Source: CAD feature listing. Evaluate the final solid. Frame: model axes, mm. A direction names the side the tool comes from. Coordinates: 2 decimals unless noted, no trailing zeros. Order: outer loops, then holes, each group sorted by start corner. A loop starts at its lowest first (then second) coordinate and runs counter-clockwise, first axis right, second up. Notation, with made-up numbers: (-36, -8) - (2, -8) arc R24 cw to (2, 2) - close; hole circle Ø4 at (62, 87.5). An arc over 180 degrees is marked (long way). One line per question, with ' | ' between items. Start each with the question number.
(1) Section A-A (z = -198.5). Return the cut outline in (x, y) (3 decimals), then the cut area to 3 significant figures.
(2) Section B-B (x = 88.5). Return the cut outline in (y, z) (3 decimals).
(3) Line query: line 1 along Z through (x, y) = (24.5, 0.5); line 2 along Z through (x, y) = (128.5, 7); line 3 along X through (y, z) = (5, -198). Output: solid intervals per line, ascending.
(4) Section C-C (y = 2). Count the separate pieces of the cut face and the enclosed holes in it, then the cut area to 3 significant figures.
(5) Draft query along Z for faces 1 (the flat face through (0, 5, -150)), 2 (the flat face through (88, 5, 0)), 3 (the cylindrical face through (19.69, 1.69, -19.59)). Return one class per face: +Z half, -Z half, draft (parallel to the pull), parting line (faces both ways), or undercut.
(6) Contact query for a flat-ended pin moving along its axis: P1, Ø4.5, axis at x = 62.357, z = -4.445, coming from the +Y side. Output: stop coordinate, or through.
(7) Access query for faces 4 (the cylindrical face through (158.11, 1.69, -19.59)), 5 (the cylindrical face through (13.05, 6.64, -13.3)), 6 (the flat face through (16, 0, -176)). Directions: +Z, -Z, +X, -X, +Y, -Y. A direction counts if a zero-diameter tool reaches every point of the face in a straight line with its end or side. Return the directions, or none.
from build123d import *

# Parameters (mm, degrees)
SKETCH1_W           = 177.8
SKETCH1_H           = 304.8
BOSS_EXTRUDE1_DEPTH = 9.525
SKETCH2_W           = 142.24
SKETCH2_H           = 269.24
CUT_EXTRUDE1_DEPTH  = 10.525
SKETCH3_R           = 2.5527
CUT_EXTRUDE2_DEPTH  = 10.525
FILLET4_R           = 6.35
CUT_EXTRUDE5_DEPTH  = 5.842
CHAMFER1_SIZE       = 0.254
FILLET5_R           = 2.54


with BuildPart() as part:
    # Sketch1 → Boss-Extrude1 (new body)
    with BuildSketch(Plane(origin=(0, 0, 0), x_dir=(1, 0, 0), z_dir=(0, 1, 0))):
        with Locations((88.9, 152.4)):
            Rectangle(SKETCH1_W, SKETCH1_H)
    extrude(amount=BOSS_EXTRUDE1_DEPTH)

    # Sketch2 → Cut-Extrude1 (cut, through all)
    with BuildSketch(Plane(origin=(0, 9.525, 0), x_dir=(1, 0, 0), z_dir=(0, 1, 0))):
        with Locations((88.9, 152.4)):
            Rectangle(SKETCH2_W, SKETCH2_H)
    extrude(amount=-CUT_EXTRUDE1_DEPTH, mode=Mode.SUBTRACT)

    # Sketch3 → Cut-Extrude2 (cut, through all)
    with BuildSketch(Plane(origin=(0, 9.525, 0), x_dir=(1, 0, 0), z_dir=(0, 1, 0))):
        with Locations((4.445, 184.15)):
            Circle(SKETCH3_R)
        with Locations((4.445, 241.3)):
            Circle(SKETCH3_R)
        with Locations((62.357, 300.355)):
            Circle(SKETCH3_R)
        with Locations((4.445, 300.355)):
            Circle(SKETCH3_R)
        with Locations((173.355, 184.15)):
            Circle(SKETCH3_R)
        with Locations((173.355, 241.3)):
            Circle(SKETCH3_R)
        with Locations((173.355, 300.355)):
            Circle(SKETCH3_R)
        with Locations((115.443, 300.355)):
            Circle(SKETCH3_R)
        with Locations((173.355, 120.65)):
            Circle(SKETCH3_R)
        with Locations((173.355, 63.5)):
            Circle(SKETCH3_R)
        with Locations((173.355, 4.445)):
            Circle(SKETCH3_R)
        with Locations((115.443, 4.445)):
            Circle(SKETCH3_R)
        with Locations((62.357, 4.445)):
            Circle(SKETCH3_R)
        with Locations((4.445, 4.445)):
            Circle(SKETCH3_R)
        with Locations((4.445, 63.5)):
            Circle(SKETCH3_R)
        with Locations((4.445, 120.65)):
            Circle(SKETCH3_R)
    extrude(amount=-CUT_EXTRUDE2_DEPTH, mode=Mode.SUBTRACT)

    # Fillet4
    fillet4_edges = [part.edges().sort_by_distance(p)[0] for p in [
        (17.78, 4.7625, -17.78),
        (17.78, 4.7625, -287.02),
        (160.02, 4.7625, -287.02),
        (160.02, 4.7625, -17.78),
    ]]
    fillet(fillet4_edges, radius=FILLET4_R)

    # Sketch7 → Cut-Extrude5 (cut)
    with BuildSketch(Plane(origin=(0, 9.525, 0), x_dir=(1, 0, 0), z_dir=(0, 1, 0))):
        with BuildLine():
            Line((8.636, 280.67), (8.636, 24.13))
            ThreePointArc((8.636, 24.13), (13.174087532, 13.174087532), (24.13, 8.636))
            Line((24.13, 8.636), (153.67, 8.636))
            ThreePointArc((153.67, 8.636), (164.625912468, 13.174087532), (169.164, 24.13))
            Line((169.164, 24.13), (169.164, 280.67))
            ThreePointArc((169.164, 280.67), (164.625912468, 291.625912468), (153.67, 296.164))
            Line((153.67, 296.164), (24.13, 296.164))
            ThreePointArc((24.13, 296.164), (13.174087532, 291.625912468), (8.636, 280.67))
        make_face()
        with BuildLine():
            Line((24.13, 17.78), (153.67, 17.78))
            ThreePointArc((153.67, 17.78), (158.160128061, 19.639871939), (160.02, 24.13))
            Line((160.02, 24.13), (160.02, 280.67))
            ThreePointArc((160.02, 280.67), (158.160128061, 285.160128061), (153.67, 287.02))
            Line((153.67, 287.02), (24.13, 287.02))
            ThreePointArc((24.13, 287.02), (19.639871939, 285.160128061), (17.78, 280.67))
            Line((17.78, 280.67), (17.78, 24.13))
            ThreePointArc((17.78, 24.13), (19.639871939, 19.639871939), (24.13, 17.78))
        make_face(mode=Mode.SUBTRACT)
    extrude(amount=-CUT_EXTRUDE5_DEPTH, mode=Mode.SUBTRACT)

    # Chamfer1
    chamfer1_edges = [part.edges().sort_by_distance(p)[0] for p in [
        (17.78, 3.683, -152.4),
        (19.639871939, 3.683, -19.639871939),
        (88.9, 3.683, -17.78),
        (158.160128061, 3.683, -19.639871939),
        (160.02, 3.683, -152.4),
        (158.160128061, 3.683, -285.160128061),
        (88.9, 3.683, -287.02),
        (19.639871939, 3.683, -285.160128061),
    ]]
    chamfer(chamfer1_edges, length=CHAMFER1_SIZE)

    # Fillet5
    fillet5_edges = [part.edges().sort_by_distance(p)[0] for p in [
        (0, 4.7625, -304.8),
        (177.8, 4.7625, -304.8),
        (177.8, 4.7625, 0),
        (0, 4.7625, 0),
    ]]
    fillet(fillet5_edges, radius=FILLET5_R)


solid = part.part
Response values:
1) outline: (0, 0) - (17.78, 0) - (17.78, 3.429) - (17.526, 3.683) - (8.636, 3.683) - (8.636, 9.525) - (0, 9.525) - close; (160.02, 0) - (177.8, 0) - (177.8, 9.525) - (169.164, 9.525) - (169.164, 3.683) - (160.274, 3.683) - (160.02, 3.429) - close | area: 232 mm²
2) outline: (0, -304.8) - (9.525, -304.8) - (9.525, -296.164) - (3.683, -296.164) - (3.683, -287.274) - (3.429, -287.02) - (0, -287.02) - close; (0, -17.78) - (3.429, -17.78) - (3.683, -17.526) - (3.683, -8.636) - (9.525, -8.636) - (9.525, 0) - (0, 0) - close
3) line 1: z = -304.8 to -287.02, -17.78 to 0 | line 2: z = -304.8 to -296.16, -8.64 to 0 | line 3: x = 0 to 8.64, 169.16 to 177.8
4) separate pieces: 1 | enclosed holes: 17 | area: 15,600 mm²
5) face 1: draft | face 2: +Z half | face 3: undercut
6) P1: passes through
7) face 4: +Y, -Y | face 5: +Y | face 6: +Z, -Z, +X, -X, -Y
